from build123d import *

# Parameters (mm, degrees)
F0_R     = 10
F1_DEPTH = 2.5
F2_R     = 12.7
F3_DEPTH = 2.5
F5_R     = 2.286
F6_DEPTH = 10.001
F7_R     = 1.25
F8_DEPTH = 10.001


with BuildPart() as f1:
    # F0 (on Right) → F1 (new body)
    with BuildSketch(Plane.YZ):
        Circle(F0_R)
    extrude(amount=F1_DEPTH)

    # F2 (on face) → F3 (join)
    with BuildSketch(Plane.YZ.offset(2.5)):
        Circle(F2_R)
    extrude(amount=F3_DEPTH)

    # F4: F1 across face


with BuildPart() as f1_1:
    add(f1.part)
    add(f1.part.mirror(Plane(origin=(0, 0, 0), x_dir=(0, 1, 0), z_dir=(-1, 0, 0))))

    # F5 (on face) → F6 (cut, through all)
    with BuildSketch(Plane.YZ.offset(5)):
        Circle(F5_R)
    extrude(amount=-F6_DEPTH, mode=Mode.SUBTRACT)

    # F7 (on face) → F8 (cut, through all)
    with BuildSketch(Plane.YZ.offset(5)):
        with Locations((0, 6.25)):
            Circle(F7_R)
        with Locations((6.25, 0)):
            Circle(F7_R)
        with Locations((0, -6.25)):
            Circle(F7_R)
        with Locations((-6.25, 0)):
            Circle(F7_R)
        with Locations((-4.419417, -4.419417)):
            Circle(F7_R)
        with Locations((4.419417, -4.419417)):
            Circle(F7_R)
        with Locations((-4.419417, 4.419417)):
            Circle(F7_R)
        with Locations((4.419417, 4.419417)):
            Circle(F7_R)
    extrude(amount=-F8_DEPTH, mode=Mode.SUBTRACT)


solid = f1_1.part
Part model, mm, in its own coordinate system. A direction names the side the tool comes from. Round coordinates to 2 decimals unless told otherwise and drop trailing zeros. Write each loop counter-clockwise with the first axis right and the second up, starting at its lowest first coordinate (ties: lowest second). Pieces come first, ordered by that corner, then holes. Notation, with made-up numbers: M 13.25,69 L 17.25,69 A15 cw 17.25,77 Z; hole C 34.5,-36 d10. An arc over 180 degrees is marked long. Return JSON: item names as keys, results as strings. Group by question number.
(1) Pin check, flat tips, straight feed: pin 1 Ø3 at (y, z) = (4.42, 4.42) entering from +X; pin 2 Ø2 at (y, z) = (-4.42, 4.42) entering from +X; pin 3 Ø1 at (x, y) = (1.5, -1) entering from +Z; pin 4 Ø6 at (x, y) = (-1, 3.5) entering from -Z. Stop position of each tip, or through.
(2) Saw through at A-A on z = 0. Write the cut outline in (x, y).
(3) Which spindle directions (+Z, -Z, +X, -X, +Y, -Y) get a long thin tool onto all of the face, cutting with end or side? Do faces 1 (the face through (-2.5, -0.1, -10.3)), 2 (the face through (0, 0, 5)). Say none if no direction does.
(4) Drill centre lines: probe 1 along Z at (x, y) = (-3.5, 0); probe 2 along Y at (x, z) = (2, -4.75); probe 3 along Z at (x, y) = (1.5, 0). Where is each one in solid material? Low to high.
(5) Saw through at C-C on y = -0.75. Write the cut outline in (x, z), then the cut area to 3 significant figures.
(6) Saw through at D-D on z = -6.25. Write the cut outline in (x, y), then the cut area to 3 significant figures.
(7) Saw through at B-B on x = -0.5. Count the separate pieces of the cut face and the enclosed holes in it, then the cut area to 3 significant figures.
(8) Two-plate mould, pull along Z, no slides. Class faces 3 (the face through (5, 3, 0)), 4 (the face through (0.04, -2.17, -9.76)), 5 (the face through (0.07, 3.17, 4.47)), 6 (the face through (0.07, -0.5, -2.23)): +Z half, -Z half, draft (parallel to the pull), parting line (faces both ways), or undercut.
Returned:
{
 "1": {"pin 1": "x = 5", "pin 2": "through", "pin 3": "z = 9.99", "pin 4": "z = -12.67"},
 "2": {"outline": "M -5,-12.7 L -2.5,-12.7 L -2.5,-10 L 2.5,-10 L 2.5,-12.7 L 5,-12.7 L 5,-7.5 L -5,-7.5 Z; M -5,-5 L 5,-5 L 5,-2.29 L -5,-2.29 Z; M -5,2.29 L 5,2.29 L 5,5 L -5,5 Z; M -5,7.5 L 5,7.5 L 5,12.7 L 2.5,12.7 L 2.5,10 L -2.5,10 L -2.5,12.7 L -5,12.7 Z"},
 "3": {"face 1": "none", "face 2": "+X, -X"},
 "4": {"probe 1": "-12.7 to -7.5, -5 to -2.29, 2.29 to 5, 7.5 to 12.7", "probe 2": "-8.8 to -5.62, -3.21 to 3.21, 5.62 to 8.8", "probe 3": "-10 to -7.5, -5 to -2.29, 2.29 to 5, 7.5 to 10"},
 "5": {"outline": "M -5,-12.68 L -2.5,-12.68 L -2.5,-9.97 L 2.5,-9.97 L 2.5,-12.68 L 5,-12.68 L 5,-7.25 L -5,-7.25 Z; M -5,-5.25 L 5,-5.25 L 5,-2.16 L -5,-2.16 Z; M -5,2.16 L 5,2.16 L 5,5.25 L -5,5.25 Z; M -5,7.25 L 5,7.25 L 5,12.68 L 2.5,12.68 L 2.5,9.97 L -2.5,9.97 L -2.5,12.68 L -5,12.68 Z", "area": "143 mm²"},
 "6": {"outline": "M -5,-11.06 L -2.5,-11.06 L -2.5,-7.81 L 2.5,-7.81 L 2.5,-11.06 L 5,-11.06 L 5,-1.25 L -5,-1.25 Z; M -5,1.25 L 5,1.25 L 5,11.06 L 2.5,11.06 L 2.5,7.81 L -2.5,7.81 L -2.5,11.06 L -5,11.06 Z", "area": "164 mm²"},
 "7": {"separate pieces": "1", "enclosed holes": "9", "area": "258 mm²"},
 "8": {"face 3": "draft", "face 4": "parting line", "face 5": "undercut", "face 6": "undercut"}
}
